Autodesk Inventor part; units mm, degrees
ref_plane "Work Plane4" through (-67.5, 9.7, -88) normal (-1, 0, 0) x (0, 0, 1)
ref_plane "Work Plane5" through (-62.5, 9.7, -88) normal (1, 0, 0) x (0, 0, -1)
ref_plane "Work Plane3" through (0, 22.5, 0) normal (0, 1, 0) x (1, 0, 0)
sketch "Sketch1" plane through (0, 0, 0) normal (0, 1, 0) x (-1, 0, 0)
  line L0 (-67.5, 75) -> (67.5, 75)
  line L1 (67.5, 75) -> (67.5, -75)
  line L2 (67.5, -75) -> (-67.5, -75)
  line L3 (-67.5, -75) -> (-67.5, 75)
  line L4 (-67.5, 75) -> (67.5, -75) construction
  line L5 (67.5, 75) -> (-67.5, -75) construction
  point P0 (0, 0)
  dimension "d0" = 135
  dimension "d1" = 150
extrude "Extrusion1" add sketch "Sketch1" along normal blind 8
sketch "Sketch3" plane through (0, 8, 0) normal (0, 1, 0) x (1, 0, 0)
  line L0 (-67.5, -75) -> (67.5, -75)
  line L1 (67.5, -75) -> (67.5, 75)
  line L2 (67.5, 75) -> (-67.5, 75)
  line L3 (-67.5, 75) -> (-67.5, -75)
  line L4 (62.5, 75) -> (62.5, -70)
  line L5 (-67.5, -75) -> (67.5, -75)
  line L6 (67.5, -75) -> (67.5, 75)
  line L7 (0, 0) -> (0, -83) construction
  line L8 (-62.5, 75) -> (-62.5, -70)
  line L9 (62.5, -70) -> (-62.5, -70)
  dimension "d4" = 5
  dimension "d5" = 5
extrude "Extrusion2" add sketch "Sketch3" along normal blind 38.7 contours L3 L2 L8 L9 L4 L1 L0
sketch "Sketch4" plane through (67.5, 0, -75) normal (0, 0, -1) x (-1, 0, 0)
  line L0 (135, 0) -> (0, 0)
  line L1 (135, 0) -> (135, 46.7)
  line L2 (130, 46.7) -> (135, 46.7)
  line L3 (130, 8) -> (130, 46.7)
  line L4 (5, 8) -> (130, 8)
  line L5 (5, 8) -> (5, 46.7)
  line L6 (0, 46.7) -> (5, 46.7)
  line L7 (0, 0) -> (0, 46.7)
  line L8 (130, 8) -> (5, 8)
  line L9 (5, 8) -> (5, 0)
  line L10 (130, 8) -> (130, 0)
  line L11 (0, 0) -> (135, 0)
  line L12 (0, 0) -> (0, 46.7)
  line L13 (5, 3) -> (130, 3)
  line L14 (5, 8) -> (130, 8)
  line L15 (5, 6) -> (130, 6)
  line L16 (5, 8) -> (0, 8)
  line L17 (135, 0) -> (0, 0)
  point P0 (67.5, 0)
  dimension "d8" = 3
  dimension "d9" = 3
extrude "Extrusion3" add sketch "Sketch4" along normal blind 20 contours L0 L10 L3 L2 L1 | L0 L9 L13 L10 | L15 L9 L4 L10 | L7 L6 L5 L16
sketch "Sketch6" plane through (67.5, 0, 75) normal (1, 0, 0) x (0, 0, -1)
  line L0 (150, 0) -> (150, 8)
  line L1 (0, 0) -> (0, 46.7)
  line L2 (150, 8) -> (170, 8)
  line L3 (0, 46.7) -> (170, 46.7)
  line L4 (170, 46.7) -> (170, 8)
  line L5 (170, 21) -> (153, 21)
  line L6 (153, 21) -> (153, 33)
  line L7 (153, 33) -> (170, 33)
  line L8 (170, 33) -> (170, 21)
  point P0 (75, 0)
  dimension "d92" = 13
  dimension "d93" = 17
  dimension "d94" = 12
fillet "Fillet1" radius 2 11 edges at (67.5, 0, 0) (67.5, 46.7, -10) (67.5, 23.35, 75) (0, 46.7, 75) (0, 0, 75) (-67.5, 46.7, -10) (-67.5, 23.35, 75) (-67.5, 0, -10) (62.5, 46.7, -12.5) (-62.5, 46.7, -12.5) (0, 46.7, 70)
ref_plane "Work Plane4" through (-67.5, 9.7, -88) normal (-1, 0, 0) x (0, 0, 1)
sketch "Sketch15" plane through (62.5, 6, -75) normal (1, 0, 0) x (0, 0, -1)
  line L0 (0, 0) -> (0, 2)
  line L1 (0, 0) -> (20, 0)
  line L2 (20, 2) -> (20, 0)
  line L3 (0, 2) -> (20, 2)
  point P0 (-75, -6)
extrude "Extrusion8" add sketch "Sketch15" along normal blind 2.5
sketch "Sketch16" plane through (0, 8, 0) normal (0, 1, 0) x (1, 0, 0)
  line L0 (-62.5, -35) -> (-46.5, -35)
  line L1 (-46.5, -35) -> (-46.5, 5)
  line L2 (-46.5, 5) -> (-62.5, 5)
  line L3 (-62.5, 5) -> (-62.5, -35)
  line L4 (62.5, -70) -> (-62.5, -70)
  line L5 (-62.5, -70) -> (-62.5, 95)
  line L6 (46.5, -70) -> (62.5, -70)
  line L7 (62.5, -70) -> (62.5, -30)
  line L8 (62.5, -30) -> (46.5, -30)
  line L9 (46.5, -30) -> (46.5, -70)
  line L10 (62.5, 95) -> (62.5, -70)
  point P0 (0, 0)
  dimension "d39" = 35
  dimension "d40" = 0
  dimension "d41" = 16
  dimension "d42" = 40
  dimension "d43" = 0
  dimension "d44" = 0
  dimension "d45" = 40
  dimension "d46" = 16
extrude "Extrusion9" add sketch "Sketch16" along normal blind 16
fillet "Fillet4" radius 1 8 edges at (46.5, 24, 50) (54.5, 24, 30) (46.5, 16, 30) (-46.5, 24, 15) (-46.5, 16, -5) (-54.5, 24, 35) (-54.5, 24, -5) (-46.5, 16, 35)
sketch "Sketch17" plane through (0, 24, 0) normal (0, 1, 0) x (1, 0, 0)
  circle A0 centre (-56.5, -25) radius 2.25
  line L0 (-62.5, -34) -> (-62.5, 4)
  line L1 (-47.5, -34) -> (-62.5, -34)
  circle A1 centre (54.5, -57.5) radius 2.25
  line L2 (47.5, -70) -> (47.5, -31)
  line L3 (47.5, -31) -> (62.5, -31)
  line L4 (62.5, -70) -> (50.5, -70)
  point P0 (0, 0)
  dimension "d50" = 4.5
  dimension "d51" = 6
  dimension "d52" = 9
  dimension "d53" = 4.5
  dimension "d54" = 7
  dimension "d90" = 12.5
extrude "Extrusion10" cut sketch "Sketch17" against normal blind 12
ref_plane "Work Plane5" through (-62.5, 9.7, -88) normal (1, 0, 0) x (0, 0, -1)
sketch "Sketch18" plane through (-62.5, 9.7, -88) normal (1, 0, 0) x (0, 0, -1)
  circle A0 centre (-58, 19) radius 2.25
  circle A1 centre (-27.2, 19) radius 2.25
  line L0 (0, 8.1) -> (0, 14.1)
  line L1 (-27.2, 19) -> (-58, 19)
  line L2 (7, 37) -> (-160, 37)
  line L3 (-158, -1.7) -> (-158, 35)
  point P0 (-88, -9.7)
  dimension "d60" = 4.5
  dimension "d61" = 4.5
  dimension "d62" = 30.8
  dimension "d67" = 100
  dimension "d91" = 18
extrude "Extrusion11" cut sketch "Sketch18" against normal through all
ref_plane "Work Plane3" through (0, 22.5, 0) normal (0, 1, 0) x (1, 0, 0)
sketch "Sketch21" plane through (0, 22.5, 0) normal (0, 1, 0) x (1, 0, 0)
  circle A0 centre (54.5, -57.5) radius 2.25
  line L0 (50.75, -55.3349) -> (54.5, -53.1699)
  line L1 (54.5, -53.1699) -> (58.25, -55.3349)
  line L2 (58.25, -55.3349) -> (58.25, -59.6651)
  line L3 (58.25, -59.6651) -> (54.5, -61.8301)
  line L4 (54.5, -61.8301) -> (50.75, -59.6651)
  line L5 (50.75, -59.6651) -> (50.75, -55.3349)
  line L6 (-62.5, -35) -> (-62.5, -70)
  line L7 (46.5, -70) -> (46.5, -31)
  circle A1 centre (-56.5, -25) radius 2.25
  line L8 (-52.75, -27.1651) -> (-56.5, -29.3301)
  line L9 (-56.5, -29.3301) -> (-60.25, -27.1651)
  line L10 (-60.25, -27.1651) -> (-60.25, -22.8349)
  line L11 (-60.25, -22.8349) -> (-56.5, -20.6699)
  line L12 (-56.5, -20.6699) -> (-52.75, -22.8349)
  line L13 (-52.75, -22.8349) -> (-52.75, -27.1651)
  point P0 (0, 0)
  dimension "d78" = 7.5
  dimension "d79" = 7.5
extrude "Extrusion13" cut sketch "Sketch21" against normal blind 3.15
extrude "Extrusion14" cut sketch "Sketch6" against normal through all
sketch "Sketch22" plane through (0, 8, 0) normal (0, 1, 0) x (1, 0, 0)
  line L0 (224, -151) -> (-256, -151)
  line L1 (-256, -151) -> (-256, 143)
  line L2 (-256, 143) -> (224, 143)
  line L3 (224, 143) -> (224, -151)
  point P0 (0, 0)
extrude "Extrusion15" cut sketch "Sketch22" along normal through all
ref_plane "Work Plane6" through (62.5, 3, -65) normal (0, 0, -1) x (-1, 0, 0)
sketch "Sketch23" plane through (62.5, 3, -65) normal (0, 0, -1) x (-1, 0, 0)
  line L0 (-63, 29) -> (227, 29)
  line L1 (227, 29) -> (227, -39)
  line L2 (227, -39) -> (-63, -39)
  line L3 (-63, -39) -> (-63, 29)
  point P0 (62.5, -3)
extrude "Extrusion16" cut sketch "Sketch23" against normal through all
properties part number "Prova supporti"
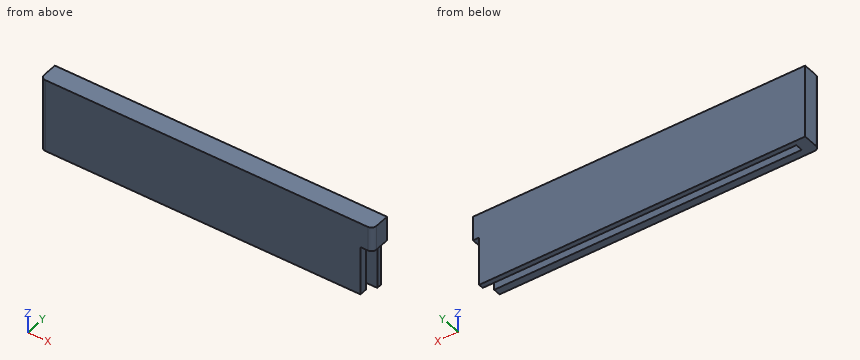
The listing builds one solid part. Answer for the finished solid, in the listing's coordinates (mm). Coordinates: 2 decimals unless noted, no trailing zeros. Write each loop counter-clockwise with the first axis right and the second up, starting at its lowest first coordinate (ties: lowest second). Pieces come first, ordered by that corner, then holes. Notation, with made-up numbers: (73, 53.25) - (92, 53.25) arc R14 cw to (92, 74.25) - close; hole circle Ø7 at (0, 9.25). An arc over 180 degrees is marked (long way). Return JSON: item names as keys, results as strings. Group by question number.
Q1. The part is cut by section A-A on x = 22.5. Write down the section's boundary in (y, z).
Q2. The part is cut by section B-B on y = 4.25. Write down the section's boundary in (x, z), and give its area (3 significant figures).
Q3. Find the intervals of material crossed by line 1 along Y through (x, z) = (38, -84.25); line 2 along X through (y, z) = (6.25, -79.75); line 3 along Z through (x, y) = (38, 3.5), in increasing order. Write a range as [from, to].
Q4. The part is cut by section C-C on z = -89.25. Write down the section's boundary in (x, y).
Q5. Flat-ended cylindrical pins translate along their axes: pin 1 Ø4 at (x, y) = (25.5, 5.5) entering from -Z; pin 2 Ø0.9 at (y, z) = (5, -87) entering from +X; pin 3 Ø2 at (y, z) = (7.5, -84) entering from +X; pin 4 Ø3.5 at (y, z) = (1.5, -87) entering from +X. Find the tip coordinate at first contact, or state that the pin passes through.
Evaluation:
{
 "1": {"outline": "(0, -95) - (3, -95) - (3, -75) - (6, -75) - (6, -95) - (8, -95) - (8, -65) - (0, -65) - close"},
 "2": {"outline": "(-67.5, -95) - (-62.5, -95) - (-62.5, -75) - (67.5, -75) - (67.5, -65) - (-67.5, -65) - close", "area": "1,450 mm2"},
 "3": {"line 1": "y = [0, 3], [6, 8]", "line 2": "x = [-67.5, 65]", "line 3": "z = [-75, -65]"},
 "4": {"outline": "(-67.5, 2) arc R2 ccw to (-65.5, 0) - (62.5, 0) - (62.5, 3) - (-62.5, 3) - (-62.5, 6) - (65, 6) - (65, 8) - (-67.5, 8) - close"},
 "5": {"pin 1": "stops at z = -95", "pin 2": "stops at x = -62.5", "pin 3": "stops at x = 65", "pin 4": "stops at x = 62.5"}
}
